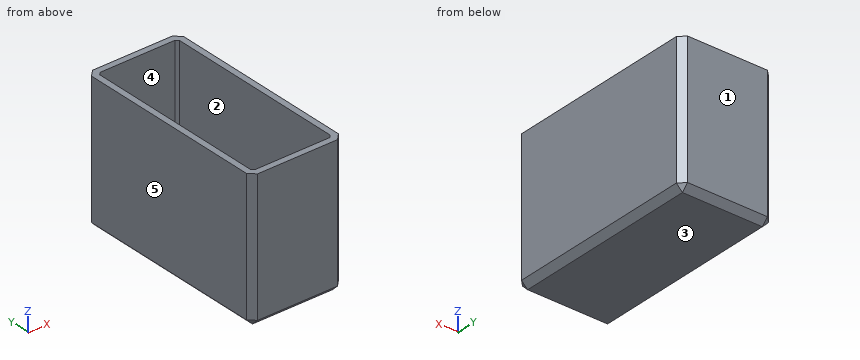
```python
from build123d import *

# Parameters (mm, degrees)
F0_W     = 30
F0_H     = 65
F1_DEPTH = 45
F2_SIZE  = 2
F3_T     = -2


with BuildPart() as f1:
    # F0 (on Top) → F1 (new body)
    with BuildSketch(Plane.XY):
        Rectangle(F0_W, F0_H)
    extrude(amount=F1_DEPTH)

    # F2
    f2_edges = [f1.edges().sort_by_distance(p)[0] for p in [
        (15, -32.5, 22.5),
        (-15, -32.5, 22.5),
        (15, 32.5, 22.5),
        (-15, 32.5, 22.5),
        (15, 0, 0),
        (-15, 0, 0),
        (0, 32.5, 0),
        (0, -32.5, 0),
    ]]
    chamfer(f2_edges, length=F2_SIZE)

    # F3
    f3_openings = [f1.faces().sort_by_distance(p)[0] for p in [
        (0, 0, 45),
    ]]
    offset(amount=F3_T, openings=f3_openings)


solid = f1.part
```
For this review, take the finished solid that the model builds, in its own axes (mm). Face numbers are marked on the shaded views. A direction names the side the tool comes from. Coordinates: 2 decimals unless noted, no trailing zeros. Write each loop counter-clockwise with the first axis right and the second up, starting at its lowest first coordinate (ties: lowest second). Pieces come first, ordered by that corner, then holes.
(1) Wall thickness on probe 1 along Y at (x, z) = (-8, 32); probe 2 along X at (y, z) = (20, 33.5); probe 3 along Z at (x, y) = (3.75, 13): over which ranges is each line inside the solid? List them lowest first.
(2) For pin 1 Ø1.5 at (x, y) = (10, 21.5) entering from +Z, flat-tipped, find the tip position at first contact; note if it passes through.
(3) Add section C-C on z = 40. Give the boundary of the cut face in (x, y), then the cut area to 3 significant figures.
(4) The part is to be moulded in two halves that separate along Y. For the marked faces 1, 2 and 3, say which applies: +Y half, -Y half, draft (parallel to the pull), parting line (faces both ways), or undercut.
(5) Add section B-B on x = -2. Give the boundary of the cut face in (y, z), then the cut area to 3 significant figures.
(6) Add section A-A on y = -16.5. Give the boundary of the cut face in (x, z), then the cut area to 3 significant figures.
(7) Tool access review of the marked faces 4 and 5: name each direction out of +Z, -Z, +X, -X, +Y, -Y from which nothing blocks a thin tool from reaching the whole face with its end or side.
Answer sheet:
1. probe 1: y = -32.5 to -30.5, 30.5 to 32.5
1. probe 2: x = -15 to -13, 13 to 15
1. probe 3: z = 0 to 2
2. pin 1: stops at z = 2
3. outline: (-15, -30.5) - (-13, -32.5) - (13, -32.5) - (15, -30.5) - (15, 30.5) - (13, 32.5) - (-13, 32.5) - (-15, 30.5) - close; hole (-13, -29.67) - (-12.17, -30.5) - (12.17, -30.5) - (13, -29.67) - (13, 29.67) - (12.17, 30.5) - (-12.17, 30.5) - (-13, 29.67) - close
3. area: 357 mm2
4. face 1: +Y half
4. face 2: undercut
4. face 3: draft
5. outline: (-32.5, 2) - (-30.5, 0) - (30.5, 0) - (32.5, 2) - (32.5, 45) - (30.5, 45) - (30.5, 2.83) - (29.67, 2) - (-29.67, 2) - (-30.5, 2.83) - (-30.5, 45) - (-32.5, 45) - close
5. area: 299 mm2
6. outline: (-15, 2) - (-13, 0) - (13, 0) - (15, 2) - (15, 45) - (13, 45) - (13, 2.83) - (12.17, 2) - (-12.17, 2) - (-13, 2.83) - (-13, 45) - (-15, 45) - close
6. area: 229 mm2
7. face 4: +Z
7. face 5: +Z, -Z, -X, +Y, -Y
